Source: CAD feature listing. Evaluate the final solid. Frame: model axes, mm. A direction names the side the tool comes from. Coordinates: 2 decimals unless noted, no trailing zeros. Loops run counter-clockwise (first coordinate to the right, second up) from the corner with the lowest first, then second, coordinate; pieces in that order, holes last.
Item 1: Line query: probe 1 along Z at (x, y) = (5.25, -17.5); probe 2 along Y at (x, z) = (7.5, 9.5) (3 decimals); probe 3 along Y at (x, z) = (6.25, 20.5). Output: solid intervals per line, ascending.
Item 2: Section query A-A, the plane y = 2. Return the cut outline in (x, z).
Item 3: Pin query (flat end, axial travel): pin 1 Ø2 at (x, z) = (9, -11) entering from +Y; pin 2 Ø2 at (x, y) = (6, 11) entering from -Z; pin 3 Ø1.5 at (x, y) = (8, -4.5) entering from +Z. Return the tip coordinate at first contact, or that it passes through.
Item 4: Pull-direction query (Z, two-part tool) for faces 4 (the cylindrical face through (7.4, -18.21, 19.25)), 5 (the cylindrical face through (7.395, -14.848, -20.846)), 6 (the flat face through (0, -16, -20)), 7 (the cylindrical face through (7.4, -24.47, -10.17)); classes: +Z half, -Z half, draft (parallel to the pull), parting line (faces both ways), or undercut.
Item 5: Reachability of faces 1 (the cylindrical face through (7.4, -21.77, -15.11)), 2 (the cylindrical face through (7.395, 21.328, -14.147)), 3 (the cylindrical face through (7.395, 25.314, 3.772)) from +Z, -Z, +X, -X, +Y, -Y: full face, straight path, thin tool, end or side. Return the list, or none.
```python
from build123d import *

# Parameters (mm, degrees)
F0_R     = 25
F1_DEPTH = 15
F3_DEPTH = 15
F4_DEPTH = 25


with BuildPart() as f1:
    # F0 (on Right) → F1 (new body)
    with BuildSketch(Plane.YZ):
        Circle(F0_R)
    extrude(amount=F1_DEPTH)

    # F2 (on Right) → F3 (join)
    with BuildSketch(Plane.YZ):
        with BuildLine():
            Line((8.7667769657, 24.0451374911), (9.167363807, 24.8638179053))
            ThreePointArc((9.167363807, 24.8638179053), (0, 26.5), (-9.167363807, 24.8638179053))
            Line((-9.167363807, 24.8638179053), (-8.7667769657, 24.0451374911))
            ThreePointArc((-8.7667769657, 24.0451374911), (-9.6126216367, 23.7196652717), (-10.4464123148, 23.3644491713))
            Line((-10.4464123148, 23.3644491713), (-10.8772899015, 24.1647380371))
            ThreePointArc((-10.8772899015, 24.1647380371), (-11.6457890541, 23.8038987838), (-12.4023348608, 23.4186269879))
            Line((-12.4023348608, 23.4186269879), (-11.9556482444, 22.6293501981))
            ThreePointArc((-11.9556482444, 22.6293501981), (-12.3825347012, 22.3986126737), (-12.804969819, 22.1598231777))
            Line((-12.804969819, 22.1598231777), (-13.3223791829, 22.9077326007))
            ThreePointArc((-13.3223791829, 22.9077326007), (-13.9672221354, 22.5203620268), (-14.600810194, 22.1148443738))
            Line((-14.600810194, 22.1148443738), (-14.015124401, 21.4149784813))
            ThreePointArc((-14.015124401, 21.4149784813), (-14.7606746545, 20.9080725815), (-15.4879088774, 20.3752225494))
            Line((-15.4879088774, 20.3752225494), (-16.2037561785, 20.9687454491))
            ThreePointArc((-16.2037561785, 20.9687454491), (-18.2372791356, 19.2263269953), (-20.0845666163, 17.2875731043))
            Line((-20.0845666163, 17.2875731043), (-19.3056392832, 16.8023006519))
            ThreePointArc((-19.3056392832, 16.8023006519), (-19.7753879115, 16.2468165583), (-20.2291590487, 15.6782058768))
            Line((-20.2291590487, 15.6782058768), (-21.0144669293, 16.1444163622))
            ThreePointArc((-21.0144669293, 16.1444163622), (-21.6282376373, 15.3123916063), (-22.2090853884, 14.4570580068))
            Line((-22.2090853884, 14.4570580068), (-21.3699018236, 14.0837605553))
            ThreePointArc((-21.3699018236, 14.0837605553), (-21.7713613337, 13.4548445182), (-22.154317385, 12.8144932219))
            Line((-22.154317385, 12.8144932219), (-22.9818096131, 13.194181555))
            ThreePointArc((-22.9818096131, 13.194181555), (-24.0639443096, 11.0984946846), (-24.9554549092, 8.9148903682))
            Line((-24.9554549092, 8.9148903682), (-24.1033509171, 8.6054337427))
            ThreePointArc((-24.1033509171, 8.6054337427), (-24.3734577278, 7.8076612198), (-24.6171678383, 7.0014329212))
            Line((-24.6171678383, 7.0014329212), (-25.4871480775, 7.2563959978))
            ThreePointArc((-25.4871480775, 7.2563959978), (-25.6948474434, 6.4826549236), (-25.8790632637, 5.7029890927))
            Line((-25.8790632637, 5.7029890927), (-25.0040927329, 5.4608023163))
            ThreePointArc((-25.0040927329, 5.4608023163), (-25.2499410388, 4.1791737064), (-25.4301414932, 2.8866795751))
            Line((-25.4301414932, 2.8866795751), (-26.3314749458, 2.9838611194))
            ThreePointArc((-26.3314749458, 2.9838611194), (-26.4345464349, -1.8613851782), (-25.6535038217, -6.6443766953))
            Line((-25.6535038217, -6.6443766953), (-24.770581207, -6.4376487942))
            ThreePointArc((-24.770581207, -6.4376487942), (-24.4413101827, -7.5925866398), (-24.0582217907, -8.7308063544))
            Line((-24.0582217907, -8.7308063544), (-24.8963284614, -9.0787019525))
            ThreePointArc((-24.8963284614, -9.0787019525), (-24.4631018107, -10.1885548434), (-23.980427863, -11.2778135961))
            Line((-23.980427863, -11.2778135961), (-23.1421674569, -10.9300091824))
            ThreePointArc((-23.1421674569, -10.9300091824), (-22.4663708469, -12.2591678469), (-21.714316209, -13.5467149858))
            Line((-21.714316209, -13.5467149858), (-22.4678164464, -14.0515915159))
            ThreePointArc((-22.4678164464, -14.0515915159), (-21.7600378171, -15.1245083953), (-21.0010668987, -16.1618436175))
            Line((-21.0010668987, -16.1618436175), (-20.2669140588, -15.6293701045))
            ThreePointArc((-20.2669140588, -15.6293701045), (-18.8785289932, -17.2808031753), (-17.3559862837, -18.809432619))
            Line((-17.3559862837, -18.809432619), (-17.9685421311, -19.4777178766))
            ThreePointArc((-17.9685421311, -19.4777178766), (-17.0517267057, -20.2851821869), (-16.0986698562, -21.0495327468))
            Line((-16.0986698562, -21.0495327468), (-15.4646276122, -20.3928984734))
            ThreePointArc((-15.4646276122, -20.3928984734), (-14.8389602034, -20.8525843821), (-14.1996376023, -21.2930812071))
            Line((-14.1996376023, -21.2930812071), (-14.7619831931, -22.0075862422))
            ThreePointArc((-14.7619831931, -22.0075862422), (-11.0464779391, -24.0878667619), (-7.0457455252, -25.5461830807))
            Line((-7.0457455252, -25.5461830807), (-6.7939183804, -24.675244444))
            ThreePointArc((-6.7939183804, -24.675244444), (-5.8600138867, -24.9135555989), (-4.9177986021, -25.1165338421))
            Line((-4.9177986021, -25.1165338421), (-5.1447925105, -25.9957902366))
            ThreePointArc((-5.1447925105, -25.9957902366), (-3.4860237826, -26.2697095185), (-1.8132238626, -26.4378936231))
            Line((-1.8132238626, -26.4378936231), (-1.8132238626, -25.5291448066))
            ThreePointArc((-1.8132238626, -25.5291448066), (-0.9071820061, -25.5773735192), (0, -25.5934564944))
            Line((0, -25.5934564944), (0, -26.5))
            ThreePointArc((0, -26.5), (7.9810933491, -25.2695894101), (15.2210529793, -21.6926150153))
            Line((15.2210529793, -21.6926150153), (14.6331353927, -20.9975323291))
            ThreePointArc((14.6331353927, -20.9975323291), (17.3553470272, -18.8100224586), (19.7544267456, -16.2722966812))
            Line((19.7544267456, -16.2722966812), (20.5165201568, -16.7726682629))
            ThreePointArc((20.5165201568, -16.7726682629), (21.1093381988, -16.0201698122), (21.6745709529, -15.2467365035))
            Line((21.6745709529, -15.2467365035), (20.9011169086, -14.7705222421))
            ThreePointArc((20.9011169086, -14.7705222421), (21.3340901742, -14.1379493481), (21.7479249086, -13.4926934858))
            Line((21.7479249086, -13.4926934858), (22.5588780332, -13.9049279712))
            ThreePointArc((22.5588780332, -13.9049279712), (23.0060041379, -13.1519494223), (23.4280063282, -12.3846081684))
            Line((23.4280063282, -12.3846081684), (22.6385053111, -11.93830359))
            ThreePointArc((22.6385053111, -11.93830359), (23.053686941, -11.1154187397), (23.4389697754, -10.2781180768))
            Line((23.4389697754, -10.2781180768), (24.267045054, -10.6470899475))
            ThreePointArc((24.267045054, -10.6470899475), (24.6102450352, -9.8278094866), (24.925794396, -8.9974870785))
            Line((24.925794396, -8.9974870785), (24.1178160427, -8.5648096686))
            ThreePointArc((24.1178160427, -8.5648096686), (24.5495291024, -7.2350284161), (24.9079826306, -5.8836567376))
            Line((24.9079826306, -5.8836567376), (25.7684601297, -6.183563903))
            ThreePointArc((25.7684601297, -6.183563903), (26.4382446614, -1.8080982335), (26.3703819824, 2.6178147571))
            Line((26.3703819824, 2.6178147571), (25.4592235001, 2.6178147571))
            ThreePointArc((25.4592235001, 2.6178147571), (25.3114799464, 3.7886670817), (25.1099187709, 4.9514638896))
            Line((25.1099187709, 4.9514638896), (25.9998556245, 5.1242079882))
            ThreePointArc((25.9998556245, 5.1242079882), (25.8404971142, 5.8752624528), (25.6594477487, 6.6213851444))
            Line((25.6594477487, 6.6213851444), (24.7804638947, 6.3995018943))
            ThreePointArc((24.7804638947, 6.3995018943), (24.565922533, 7.179168854), (24.3268571199, 7.9516688812))
            Line((24.3268571199, 7.9516688812), (25.1932767406, 8.2188081296))
            ThreePointArc((25.1932767406, 8.2188081296), (24.9270062981, 8.9941290304), (24.6368818038, 9.7608429444))
            Line((24.6368818038, 9.7608429444), (23.797443763, 9.4184226747))
            ThreePointArc((23.797443763, 9.4184226747), (23.3599091422, 10.4565606294), (22.8771127008, 11.4744381042))
            Line((22.8771127008, 11.4744381042), (23.7017475478, 11.8523062389))
            ThreePointArc((23.7017475478, 11.8523062389), (22.0684810977, 14.6707921409), (20.1017465557, 17.2675935038))
            Line((20.1017465557, 17.2675935038), (19.3490827507, 16.752253939))
            ThreePointArc((19.3490827507, 16.752253939), (16.9830440824, 19.1468333942), (14.3231931258, 21.2101662891))
            Line((14.3231931258, 21.2101662891), (14.767734035, 22.0037276722))
            ThreePointArc((14.767734035, 22.0037276722), (13.3677835034, 22.8812666652), (11.915866869, 23.6698567119))
            Line((11.915866869, 23.6698567119), (11.86207115, 23.5452761594))
            Line((11.86207115, 23.5452761594), (11.5231473656, 22.8526167019))
            ThreePointArc((11.5231473656, 22.8526167019), (10.1624693751, 23.4893429353), (8.7667769657, 24.0451374911))
        make_face()
        with BuildLine():
            ThreePointArc((25, 0), (-11.1699631634, -22.3658651281), (-15.0185538343, 19.9860711678))
            ThreePointArc((-15.0185538343, 19.9860711678), (-13.7681439239, 20.8671563202), (-12.4661896956, 21.6701203152))
            ThreePointArc((-12.4661896956, 21.6701203152), (-0.6839357102, 24.9906428878), (11.262295833, 22.3195137171))
            ThreePointArc((11.262295833, 22.3195137171), (21.2903428322, 13.1042474827), (25, 0))
        make_face(mode=Mode.SUBTRACT)
    extrude(amount=F3_DEPTH)

    # F2 (on Right) → F4 (cut)
    with BuildSketch(Plane.YZ):
        with BuildLine():
            ThreePointArc((-12.4661896956, 21.6701203152), (-13.7681439239, 20.8671563202), (-15.0185538343, 19.9860711678))
            ThreePointArc((-15.0185538343, 19.9860711678), (-11.1699631634, -22.3658651281), (25, 0))
            ThreePointArc((25, 0), (21.2903428322, 13.1042474827), (11.262295833, 22.3195137171))
            ThreePointArc((11.262295833, 22.3195137171), (-0.6839357102, 24.9906428878), (-12.4661896956, 21.6701203152))
        make_face()
    extrude(amount=F4_DEPTH, mode=Mode.SUBTRACT)


solid = f1.part
```
Verdict:
1. probe 1: z = -19.9 to -18.97, -18.68 to -17.85, 17.85 to 19.9
1. probe 2: y = -24.739 to -23.125, 23.125 to 23.765, 23.997 to 24.739
1. probe 3: y = -16.79 to -15.64, -15.32 to -14.31, 14.31 to 15.32
2. outline: (0, -26.42) - (15, -26.42) - (15, -24.92) - (0, -24.92) - close; (0, 24.92) - (15, 24.92) - (15, 26.42) - (0, 26.42) - close
3. pin 1: stops at y = 24.54
3. pin 2: stops at z = -24.54
3. pin 3: stops at z = 26.23
4. face 4: +Z half
4. face 5: undercut
4. face 6: draft
4. face 7: -Z half
5. face 1: -Z, +X, -X, -Y
5. face 2: +X, -X
5. face 3: +X, -X, +Y
